Geometry: final body of the model. Coordinates: model frame, mm. Give positions to 0.01 mm unless a question says otherwise; leave off trailing zeros. Write each loop counter-clockwise with the first axis right and the second up, starting at its lowest first coordinate (ties: lowest second). Pieces come first, ordered by that corner, then holes. Notation, with made-up numbers: (1, 86) - (49, 86) arc R26 ccw to (49, 115) - close; hole circle Ø3 at (-38, -19). An arc over 180 degrees is marked (long way). Return JSON: item names as keys, results as strings.
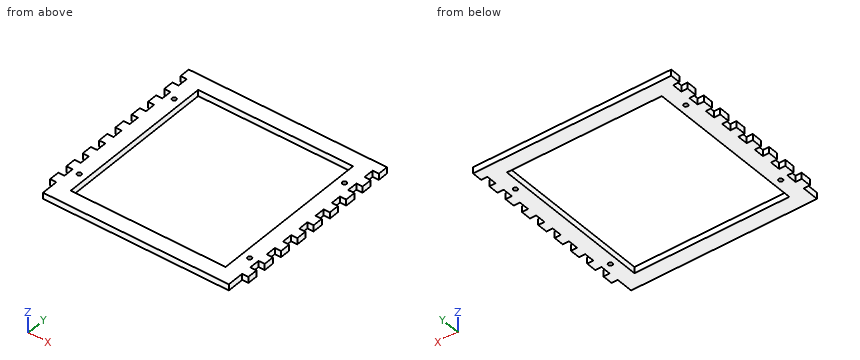
Autodesk Inventor part; units mm, degrees
ref_plane "YZ Plane" through (0, 0, 0) normal (1, 0, 0) x (0, 1, 0)
ref_plane "XZ Plane" through (0, 0, 0) normal (0, 1, 0) x (-1, 0, 0)
ref_plane "XY Plane" through (0, 0, 0) normal (0, 0, 1) x (1, 0, 0)
sketch "Эскиз1" plane through (0, 0, 0) normal (0, 0, 1) x (1, 0, 0)
  line L0 (0, 20) -> (0, 30)
  line L1 (0, 20) -> (6, 20)
  line L2 (6, 30) -> (6, 20)
  line L3 (0, 30) -> (6, 30)
  line L4 (0, 0) -> (0, 10)
  line L5 (0, 0) -> (6, 0)
  line L6 (6, 10) -> (6, 0)
  line L7 (0, 10) -> (6, 10)
  line L8 (0, -20) -> (0, -10)
  line L9 (0, -20) -> (6, -20)
  line L10 (6, -10) -> (6, -20)
  line L11 (0, -10) -> (6, -10)
  line L12 (0, -40) -> (0, -30)
  line L13 (0, -40) -> (6, -40)
  line L14 (6, -30) -> (6, -40)
  line L15 (0, -30) -> (6, -30)
  line L16 (0, -60) -> (0, -50)
  line L17 (0, -60) -> (6, -60)
  line L18 (6, -50) -> (6, -60)
  line L19 (0, -50) -> (6, -50)
  line L20 (0, -80) -> (0, -70)
  line L21 (0, -80) -> (6, -80)
  line L22 (6, -70) -> (6, -80)
  line L23 (0, -70) -> (6, -70)
  line L24 (0, -100) -> (0, -90)
  line L25 (0, -100) -> (6, -100)
  line L26 (6, -90) -> (6, -100)
  line L27 (0, -90) -> (6, -90)
  line L28 (0, -120) -> (0, -110)
  line L29 (0, -120) -> (6, -120)
  line L30 (6, -110) -> (6, -120)
  line L31 (0, -110) -> (6, -110)
  line L32 (0, -140) -> (0, -130)
  line L33 (0, -140) -> (6, -140)
  line L34 (6, -130) -> (6, -140)
  line L35 (0, -130) -> (6, -130)
  line L36 (0, -156.3478) -> (0, -140)
  line L37 (-180, -140) -> (-180, -156.3478)
  line L38 (-186, -140) -> (-186, -130)
  line L39 (-186, -140) -> (-180, -140)
  line L40 (-180, -130) -> (-180, -140)
  line L41 (-186, -130) -> (-180, -130)
  line L42 (-186, -120) -> (-186, -110)
  line L43 (-186, -120) -> (-180, -120)
  line L44 (-180, -110) -> (-180, -120)
  line L45 (-186, -110) -> (-180, -110)
  line L46 (-186, -100) -> (-186, -90)
  line L47 (-186, -100) -> (-180, -100)
  line L48 (-180, -90) -> (-180, -100)
  line L49 (-186, -90) -> (-180, -90)
  line L50 (-186, -80) -> (-186, -70)
  line L51 (-186, -80) -> (-180, -80)
  line L52 (-180, -70) -> (-180, -80)
  line L53 (-186, -70) -> (-180, -70)
  line L54 (-186, -60) -> (-186, -50)
  line L55 (-186, -60) -> (-180, -60)
  line L56 (-180, -50) -> (-180, -60)
  line L57 (-186, -50) -> (-180, -50)
  line L58 (-186, -40) -> (-186, -30)
  line L59 (-186, -40) -> (-180, -40)
  line L60 (-180, -30) -> (-180, -40)
  line L61 (-186, -30) -> (-180, -30)
  line L62 (-186, 20) -> (-186, 30)
  line L63 (-186, 20) -> (-180, 20)
  line L64 (-180, 30) -> (-180, 20)
  line L65 (-186, 30) -> (-180, 30)
  line L66 (-186, 0) -> (-186, 10)
  line L67 (-186, 0) -> (-180, 0)
  line L68 (-180, 10) -> (-180, 0)
  line L69 (-186, 10) -> (-180, 10)
  line L70 (-186, -20) -> (-186, -10)
  line L71 (-186, -20) -> (-180, -20)
  line L72 (-180, -10) -> (-180, -20)
  line L73 (-186, -10) -> (-180, -10)
  line L74 (0, -156.3478) -> (-180, -156.3478)
  line L75 (-180, -156.3478) -> (-180, 30)
  line L76 (-180, 30) -> (0, 30)
  line L77 (0, 30) -> (0, -156.3478)
extrude "Выдавливание1" add sketch "Эскиз1" along normal blind 6
sketch "Эскиз2" plane through (0, 0, 6) normal (0, 0, 1) x (1, 0, 0)
  line L0 (-15, 15) -> (-165, 15)
  line L1 (-165, 15) -> (-165, -141.3478)
  line L2 (-165, -141.3478) -> (-15, -141.3478)
  line L3 (-15, -141.3478) -> (-15, 15)
  line L4 (-186, 10) -> (-186, 0)
  line L5 (-186, 0) -> (-180, 0)
  line L6 (-180, 0) -> (-180, -10)
  line L7 (-180, -10) -> (-186, -10)
  line L8 (-186, -10) -> (-186, -20)
  line L9 (-186, -20) -> (-180, -20)
  line L10 (-180, -20) -> (-180, -30)
  line L11 (-180, -30) -> (-186, -30)
  line L12 (-186, -30) -> (-186, -40)
  line L13 (-186, -40) -> (-180, -40)
  line L14 (-180, -40) -> (-180, -50)
  line L15 (-180, -50) -> (-186, -50)
  line L16 (-186, -50) -> (-186, -60)
  line L17 (-186, -60) -> (-180, -60)
  line L18 (-180, -60) -> (-180, -70)
  line L19 (-180, -70) -> (-186, -70)
  line L20 (-186, -70) -> (-186, -80)
  line L21 (-186, -80) -> (-180, -80)
  line L22 (-180, -80) -> (-180, -90)
  line L23 (-180, -90) -> (-186, -90)
  line L24 (-186, -90) -> (-186, -100)
  line L25 (-186, -100) -> (-180, -100)
  line L26 (-180, -100) -> (-180, -110)
  line L27 (-180, -110) -> (-186, -110)
  line L28 (-186, -110) -> (-186, -120)
  line L29 (-186, -120) -> (-180, -120)
  line L30 (-180, -120) -> (-180, -130)
  line L31 (-180, -130) -> (-186, -130)
  line L32 (-186, -130) -> (-186, -140)
  line L33 (-186, -140) -> (-180, -140)
  line L34 (-180, -140) -> (-180, -156.3478)
  line L35 (-180, -156.3478) -> (0, -156.3478)
  line L36 (0, -156.3478) -> (0, -140)
  line L37 (0, -140) -> (6, -140)
  line L38 (6, -140) -> (6, -130)
  line L39 (6, -130) -> (0, -130)
  line L40 (0, -130) -> (0, -120)
  line L41 (0, -120) -> (6, -120)
  line L42 (6, -120) -> (6, -110)
  line L43 (6, -110) -> (0, -110)
  line L44 (0, -110) -> (0, -100)
  line L45 (0, -100) -> (6, -100)
  line L46 (6, -100) -> (6, -90)
  line L47 (6, -90) -> (0, -90)
  line L48 (0, -90) -> (0, -80)
  line L49 (0, -80) -> (6, -80)
  line L50 (6, -80) -> (6, -70)
  line L51 (6, -70) -> (0, -70)
  line L52 (0, -70) -> (0, -60)
  line L53 (0, -60) -> (6, -60)
  line L54 (6, -60) -> (6, -50)
  line L55 (6, -50) -> (0, -50)
  line L56 (0, -50) -> (0, -40)
  line L57 (0, -40) -> (6, -40)
  line L58 (6, -40) -> (6, -30)
  line L59 (6, -30) -> (0, -30)
  line L60 (0, -30) -> (0, -20)
  line L61 (0, -20) -> (6, -20)
  line L62 (6, -20) -> (6, -10)
  line L63 (6, -10) -> (0, -10)
  line L64 (0, -10) -> (0, 0)
  line L65 (0, 0) -> (6, 0)
  line L66 (6, 0) -> (6, 10)
  line L67 (6, 10) -> (0, 10)
  line L68 (0, 10) -> (0, 20)
  line L69 (0, 20) -> (6, 20)
  line L70 (6, 20) -> (6, 30)
  line L71 (6, 30) -> (-186, 30)
  line L72 (-186, 30) -> (-186, 20)
  line L73 (-186, 20) -> (-180, 20)
  line L74 (-180, 20) -> (-180, 10)
  line L75 (-180, 10) -> (-186, 10)
  dimension "d2" = 15
  dimension "d3" = 15
  dimension "d4" = 15
  dimension "d5" = 15
extrude "Выдавливание2" cut sketch "Эскиз2" against normal blind 6 contours L3 L2 L1 L0
sketch "Эскиз3" plane through (0, 0, 6) normal (0, 0, 1) x (1, 0, 0)
  circle A0 centre (-172.5, -121.3478) radius 2
  line L0 (-165, -141.3478) -> (-165, 15)
  line L1 (-165, 15) -> (-15, 15)
  line L2 (-15, 15) -> (-15, -141.3478)
  line L3 (-15, -141.3478) -> (-165, -141.3478)
  line L4 (-186, 10) -> (-186, 0)
  line L5 (-186, 0) -> (-180, 0)
  line L6 (-180, 0) -> (-180, -10)
  line L7 (-180, -10) -> (-186, -10)
  line L8 (-186, -10) -> (-186, -20)
  line L9 (-186, -20) -> (-180, -20)
  line L10 (-180, -20) -> (-180, -30)
  line L11 (-180, -30) -> (-186, -30)
  line L12 (-186, -30) -> (-186, -40)
  line L13 (-186, -40) -> (-180, -40)
  line L14 (-180, -40) -> (-180, -50)
  line L15 (-180, -50) -> (-186, -50)
  line L16 (-186, -50) -> (-186, -60)
  line L17 (-186, -60) -> (-180, -60)
  line L18 (-180, -60) -> (-180, -70)
  line L19 (-180, -70) -> (-186, -70)
  line L20 (-186, -70) -> (-186, -80)
  line L21 (-186, -80) -> (-180, -80)
  line L22 (-180, -80) -> (-180, -90)
  line L23 (-180, -90) -> (-186, -90)
  line L24 (-186, -90) -> (-186, -100)
  line L25 (-186, -100) -> (-180, -100)
  line L26 (-180, -100) -> (-180, -110)
  line L27 (-180, -110) -> (-186, -110)
  line L28 (-186, -110) -> (-186, -120)
  line L29 (-186, -120) -> (-180, -120)
  line L30 (-180, -120) -> (-180, -130)
  line L31 (-180, -130) -> (-186, -130)
  line L32 (-186, -130) -> (-186, -140)
  line L33 (-186, -140) -> (-180, -140)
  line L34 (-180, -140) -> (-180, -156.3478)
  line L35 (-180, -156.3478) -> (0, -156.3478)
  line L36 (0, -156.3478) -> (0, -140)
  line L37 (0, -140) -> (6, -140)
  line L38 (6, -140) -> (6, -130)
  line L39 (6, -130) -> (0, -130)
  line L40 (0, -130) -> (0, -120)
  line L41 (0, -120) -> (6, -120)
  line L42 (6, -120) -> (6, -110)
  line L43 (6, -110) -> (0, -110)
  line L44 (0, -110) -> (0, -100)
  line L45 (0, -100) -> (6, -100)
  line L46 (6, -100) -> (6, -90)
  line L47 (6, -90) -> (0, -90)
  line L48 (0, -90) -> (0, -80)
  line L49 (0, -80) -> (6, -80)
  line L50 (6, -80) -> (6, -70)
  line L51 (6, -70) -> (0, -70)
  line L52 (0, -70) -> (0, -60)
  line L53 (0, -60) -> (6, -60)
  line L54 (6, -60) -> (6, -50)
  line L55 (6, -50) -> (0, -50)
  line L56 (0, -50) -> (0, -40)
  line L57 (0, -40) -> (6, -40)
  line L58 (6, -40) -> (6, -30)
  line L59 (6, -30) -> (0, -30)
  line L60 (0, -30) -> (0, -20)
  line L61 (0, -20) -> (6, -20)
  line L62 (6, -20) -> (6, -10)
  line L63 (6, -10) -> (0, -10)
  line L64 (0, -10) -> (0, 0)
  line L65 (0, 0) -> (6, 0)
  line L66 (6, 0) -> (6, 10)
  line L67 (6, 10) -> (0, 10)
  line L68 (0, 10) -> (0, 20)
  line L69 (0, 20) -> (6, 20)
  line L70 (6, 20) -> (6, 30)
  line L71 (6, 30) -> (-186, 30)
  line L72 (-186, 30) -> (-186, 20)
  line L73 (-186, 20) -> (-180, 20)
  line L74 (-180, 20) -> (-180, 10)
  line L75 (-180, 10) -> (-186, 10)
  circle A1 centre (-172.5, -5) radius 2
  circle A2 centre (-7.5, -5) radius 2
  circle A3 centre (-7.5, -121.3478) radius 2
  dimension "d8" = 4
  dimension "d9" = 20
  dimension "d10" = 15
  dimension "d11" = 7.5
  dimension "d12" = 4
  dimension "d13" = 20
  dimension "d14" = 7.5
  dimension "d15" = 4
  dimension "d16" = 4
  dimension "d17" = 20
  dimension "d18" = 20
  dimension "d19" = 7.5
  dimension "d20" = 7.5
extrude "Выдавливание3" cut sketch "Эскиз3" against normal blind 10 contours A0 | A1 | A2 | A3
equation "\"d13\" = d9"
equation "\"d19\" = d11"
equation "\"d20\" = d19"
properties part number "верх"
Q1. Section query A-A, the plane y = 7.5. Return the cut outline in (x, z).
Answer key:
{"outline": "(-186, 0) - (-165, 0) - (-165, 6) - (-186, 6) - close; (-15, 0) - (6, 0) - (6, 6) - (-15, 6) - close"}
Q2. Material intervals for probe 1 along Y at (x, z) = (-7.5, 1.45); probe 2 along Y at (x, z) = (-32.5, 4.15); probe 3 along X at (y, z) = (-25, 4.15), sorted ascending. Write a range as [from, to].
Answer key:
{"probe 1": "y = [-156.35, -123.35], [-119.35, -7], [-3, 30]", "probe 2": "y = [-156.35, -141.35], [15, 30]", "probe 3": "x = [-180, -165], [-15, 0]"}
Q3. Section query B-B, the plane x = -99. Return the cut outline in (y, z), plus the area to 3 significant figures.
Answer key:
{"outline": "(-156.35, 0) - (-141.35, 0) - (-141.35, 6) - (-156.35, 6) - close; (15, 0) - (30, 0) - (30, 6) - (15, 6) - close", "area": "180 mm^2"}
Q4. Pin query (flat end, axial travel): P1, Ø1.8, axis at y = -42.5, z = 1.5, coming from the -X side; P2, Ø3, axis at y = -24.5, z = 3.5, coming from the +X side; P3, Ø3, axis at x = -182.5, z = 2.5, coming from the -Y side. Return the tip coordinate at first contact, or that it passes through.
Answer key:
{"P1": "stops at x = -180", "P2": "stops at x = 0", "P3": "stops at y = -140"}
Q5. Section query C-C, the plane z = 2. Count the separate pieces of the cut face and the enclosed holes in it, plus the area to 3 significant figures.
Answer key:
{"separate pieces": "1", "enclosed holes": "5", "area": "11,100 mm^2"}
